Part model, mm, in its own coordinate system. Face numbers are marked on the shaded views. A direction names the side the tool comes from. Round coordinates to 2 decimals unless told otherwise and drop trailing zeros. Order: outer loops, then holes, each group sorted by start corner. A loop starts at its lowest first (then second) coordinate and runs counter-clockwise, first axis right, second up. Notation, with made-up numbers: (20.5, 29.25) - (25.5, 29.25) arc R21 cw to (25.5, 36.25) - close; hole circle Ø8 at (42, -26). An arc over 180 degrees is marked (long way). Return JSON: item names as keys, results as strings. Group by question number.
Item 1: Saw through at D-D on x = 16. State how many separate pieces and enclosed holes the cut face has, and give its area (3 significant figures).
Item 2: Tool access for the marked faces 1 and 2: list every direction of +Z, -Z, +X, -X, +Y, -Y with a clear straight run to the whole face (end or side of a thin tool).
Item 3: Two-plate mould, pull along Y, no slides. Class the marked faces 3, 4 and 5: released by +Y, released by -Y, zero draft, split by the parting line, or undercut.
Item 4: Saw through at C-C on y = -32. List the corners of the cut face in (x, z) (3 decimals), and give its area (3 significant figures).
Item 5: Drop flat-ended pins along their axis: pin 1 (4.5 mm diameter, centred on x = -39.9, z = 60.66, fed in from +Y); pin 2 (2 mm diameter, centred on x = -7, y = -31.5, fed in from -Z); pin 3 (3.5 mm diameter, centred on x = -39.89, z = 60.7, fed in from +Y); pin 4 (5 mm diameter, centred on y = -32.5, z = -27, fed in from -X). Give the stop position or say it passes through.
Item 6: Saw through at B-B on x = -93. List the corners of the cut face in (y, z).
Item 7: Probe probe 1 along Y at (x, z) = (64.5, 7); probe 2 along Y at (x, z) = (20, 51.5); probe 3 along Z at (x, y) = (56, -29.5). List the from-to ranges inside material, lowest first.
Item 8: Saw through at A-A on z = 0. List the corners of the cut face in (x, y).
```python
from build123d import *

# Parameters (mm, degrees)
SKETCH_R        = 55
PAD_DEPTH       = 40
PAD_DEPTH_BACK  = 20
POCKET_DEPTH    = 33
POCKET001_START = -3
POCKET001_DEPTH = 22.5
CHAMFER_SIZE    = 7
CHAMFER001_SIZE = 4
CHAMFER002_SIZE = 6
CHAMFER003_SIZE = 2
SKETCH006_R     = 1.45
POCKET002_DEPTH = 32
SKETCH007_R     = 2
POCKET003_DEPTH = 20


with BuildPart() as part:
    # Sketch → Pad (new body, two sides)
    with BuildSketch(Plane.XZ) as pad_sk:
        with BuildLine():
            Line((-120, 75), (0, 75))
            ThreePointArc((-74.66808, -7.048245), (55.468993, -50.479608), (0, 75))
            ThreePointArc((-74.66808, -7.048245), (-83.30852, 13.959176), (-102.203647, 26.566441))
            ThreePointArc((-120, 50.506104), (-115.063539, 35.591198), (-102.203647, 26.566441))
            Line((-120, 75), (-120, 50.506104))
        make_face()
        Circle(SKETCH_R, mode=Mode.SUBTRACT)
    extrude(amount=PAD_DEPTH)
    extrude(pad_sk.sketch, amount=-PAD_DEPTH_BACK)

    # Sketch001 (on Face7 of Pad) → Pocket (cut)
    with BuildSketch(Plane(origin=(0, 20, 0), x_dir=(1, 0, 0), z_dir=(0, 1, 0))):
        with BuildLine():
            Line((54.928753, -26.568443), (75.942328, -51.611447))
            ThreePointArc((75.942328, -51.611447), (26.999321, 87.761127), (-91.820361, 0))
            Line((-211.758942, -107.924309), (-91.820361, 0))
            Line((-30.973335, -107.924309), (-211.758942, -107.924309))
            Line((-16.47613, -75.395136), (-30.973335, -107.924309))
            Line((-52.401144, -75.395136), (-16.47613, -75.395136))
            Line((-42.243927, -45.896434), (-52.401144, -75.395136))
            ThreePointArc((-31.672581, -44.331432), (-37.184839, -43.583386), (-42.243927, -45.896434))
            Line((43.621241, -30.505082), (-31.672581, -44.331432))
            Line((47.528801, -26.356267), (43.621241, -30.505082))
            ThreePointArc((54.928753, -26.568443), (51.276407, -24.801164), (47.528801, -26.356267))
        make_face()
    extrude(amount=-POCKET_DEPTH, mode=Mode.SUBTRACT)

    # Sketch003 (on Face2 of Pocket) → Pocket001 (cut)
    with BuildSketch(Plane(origin=(0, -13, 0), x_dir=(1, 0, 0), z_dir=(0, 1, 0)).offset(POCKET001_START)):
        with BuildLine():
            ThreePointArc((0, -71), (66.914561, -23.736924), (44.742136, 55.128407))
            Line((44.742136, 55.128407), (-20.564905, 108.131508))
            Line((-20.564905, 108.131508), (-158.301559, 56.449516))
            Line((-158.301559, 56.449516), (-204.416763, -71.809135))
            Line((-204.416763, -71.809135), (0, -71))
        make_face()
    extrude(amount=-POCKET001_DEPTH, mode=Mode.SUBTRACT)

    # Chamfer
    chamfer_edges = [part.edges().sort_by_distance(p)[0] for p in [
        (59.765906, -13, 32.333137),
    ]]
    chamfer(chamfer_edges, length=CHAMFER_SIZE)

    # Chamfer001
    chamfer001_edges = [part.edges().sort_by_distance(p)[0] for p in [
        (-42.243927, 3.5, 45.896434),
        (-38.03091, -13, 43.746161),
        (-47.254507, -13, 60.448217),
    ]]
    chamfer(chamfer001_edges, length=CHAMFER001_SIZE)

    # Chamfer002
    chamfer002_edges = [part.edges().sort_by_distance(p)[0] for p in [
        (66.914561, -16, 23.736924),
    ]]
    chamfer(chamfer002_edges, length=CHAMFER002_SIZE)

    # Chamfer003
    chamfer003_edges = [part.edges().sort_by_distance(p)[0] for p in [
        (-60, -38.5, 71.237496),
    ]]
    chamfer(chamfer003_edges, length=CHAMFER003_SIZE)

    # Sketch006 → Pocket002 (cut)
    with BuildSketch(Plane(origin=(0, 20, 0), x_dir=(1, 0, 0), z_dir=(0, 1, 0))):
        with Locations((-39.891945, -60.695583)):
            Circle(SKETCH006_R)
        with Locations((0.518637, -64.736641)):
            Circle(SKETCH006_R)
        with Locations((26.400654, -58.963699)):
            Circle(SKETCH006_R)
        with Locations((54.206989, -34.71735)):
            Circle(SKETCH006_R)
    extrude(amount=-POCKET002_DEPTH, mode=Mode.SUBTRACT)

    # Sketch007 → Pocket003 (cut)
    with BuildSketch(Plane(origin=(0, 20, 0), x_dir=(1, 0, 0), z_dir=(0, 1, 0))):
        with Locations((-39.904575, -60.661716)):
            Circle(SKETCH007_R)
        with Locations((0.50043, -64.755608)):
            Circle(SKETCH007_R)
        with Locations((26.37031, -58.932541)):
            Circle(SKETCH007_R)
        with Locations((54.224796, -34.742435)):
            Circle(SKETCH007_R)
    extrude(amount=-POCKET003_DEPTH, mode=Mode.SUBTRACT)


solid = part.part
```
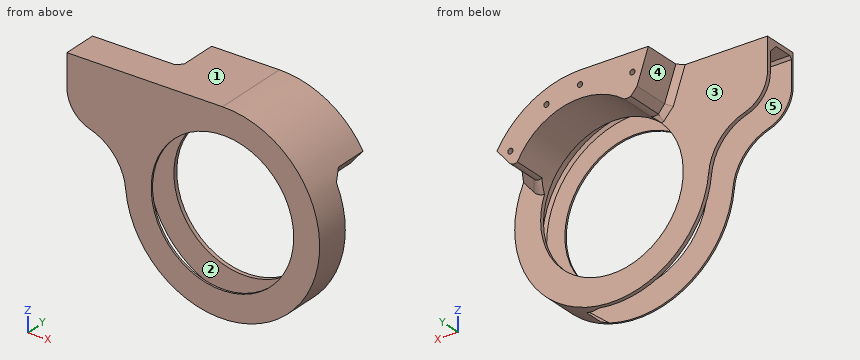
Filled in:
{
 "1": {"separate pieces": "3", "enclosed holes": "0", "area": "983 mm^2"},
 "2": {"face 1": "+Z, +X, -X, +Y, -Y", "face 2": "-X"},
 "3": {"face 3": "released by +Y", "face 4": "zero draft", "face 5": "undercut"},
 "4": {"outline": "(-120, 71.475) - (0, 71) arc R71 cw to (44.742, -55.128) - (25.978, -70.357) arc R75 ccw to (0, 75) - (-120, 75) - close", "area": "1,230 mm^2"},
 "5": {"pin 1": "stops at y = 20", "pin 2": "stops at z = 71.02", "pin 3": "stops at y = 0", "pin 4": "stops at x = 64.58"},
 "6": {"outline": "(-40, 22.43) - (-38.5, 22.43) - (-38.5, 69.37) - (-36.5, 71.37) - (-22, 71.37) - (-16, 65.37) - (-16, 22.43) - (-13, 22.43) - (-13, 75) - (-40, 75) - close"},
 "7": {"probe 1": "y = -40 to -38.5, -16 to -13", "probe 2": "y = -40 to -38.5, -16 to 20", "probe 3": "z = -49.89 to -43.65, 43.65 to 49.89"},
 "8": {"outline": "(-76, -40) - (-55, -40) - (-55, -38.5) - (-76, -38.5) - close; (-76, -16) - (-55, -16) - (-55, -13) - (-76, -13) - close; (55, -40) - (75, -40) - (75, -13) - (55, -13) - (55, -16) - (65, -16) - (71, -22) - (71, -36.5) - (69, -38.5) - (55, -38.5) - close"}
}
